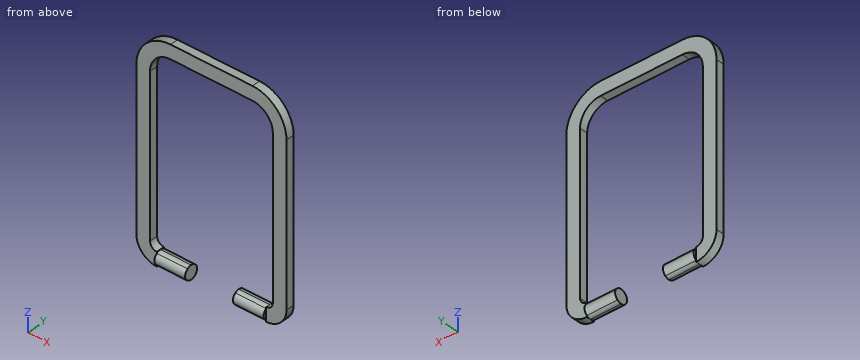
from build123d import *
from build123d import SkipClean  # not in build123d's __all__

# Parameters (mm, degrees)
F1_DEPTH = 1.2
F3_DEPTH = 4.5
F4_DEPTH = 4.5
F6_DEPTH = 4.5
F7_DEPTH = 4.5


with BuildPart() as f1:
    # F0 (on Front) → F1 (new body)
    with BuildSketch(Plane.XZ):
        with BuildLine():
            Line((4.75, 0), (-7.25, 0))
            ThreePointArc((-7.25, 0), (-10.7855339059, -1.4644660941), (-12.25, -5))
            Line((-12.25, -5), (-12.25, -28))
            ThreePointArc((-12.25, -28), (-11.3713203436, -30.1213203436), (-9.25, -31))
            Line((-9.25, -31), (-4.75, -31))
            Line((-4.75, -31), (-4.75, -29))
            Line((-4.75, -29), (-9.25, -29))
            ThreePointArc((-9.25, -29), (-9.9571067812, -28.7071067812), (-10.25, -28))
            Line((-10.25, -28), (-10.25, -5))
            ThreePointArc((-10.25, -5), (-9.3713203436, -2.8786796564), (-7.25, -2))
            Line((-7.25, -2), (4.75, -2))
            ThreePointArc((4.75, -2), (6.8713203436, -2.8786796564), (7.75, -5))
            Line((7.75, -5), (7.75, -28))
            ThreePointArc((7.75, -28), (7.4571067812, -28.7071067812), (6.75, -29))
            Line((6.75, -29), (2.25, -29))
            Line((2.25, -29), (2.25, -31))
            Line((2.25, -31), (6.75, -31))
            ThreePointArc((6.75, -31), (8.8713203436, -30.1213203436), (9.75, -28))
            Line((9.75, -28), (9.75, -5))
            ThreePointArc((9.75, -5), (8.2855339059, -1.4644660941), (4.75, 0))
        make_face()
    extrude(amount=F1_DEPTH)

    # F2 (on face) → F3 (join)
    with BuildSketch(Plane.YZ.offset(-4.75)):
        with BuildLine():
            Line((-1.2, -30.8), (-1.2, -29.2))
            ThreePointArc((-1.2, -29.2), (-1.6, -30), (-1.2, -30.8))
        make_face()
        with BuildLine():
            ThreePointArc((-0.6, -29), (-0.916227766, -29.0513167019), (-1.2, -29.2))
            Line((-1.2, -29.2), (-1.2, -30.8))
            ThreePointArc((-1.2, -30.8), (-0.916227766, -30.9486832981), (-0.6, -31))
            ThreePointArc((-0.6, -31), (-0.283772234, -30.9486832981), (0, -30.8))
            Line((0, -30.8), (0, -29.2))
            ThreePointArc((0, -29.2), (-0.283772234, -29.0513167019), (-0.6, -29))
        make_face()
        with BuildLine():
            ThreePointArc((0.4, -30), (0.294427191, -29.5527864045), (0, -29.2))
            Line((0, -29.2), (0, -30.8))
            ThreePointArc((0, -30.8), (0.294427191, -30.4472135955), (0.4, -30))
        make_face()
    extrude(amount=-F3_DEPTH)

    # F2 (on face) → F4 (cut)
    with BuildSketch(Plane.YZ.offset(-4.75)):
        with BuildLine():
            Line((0, -29), (-0.6, -29))
            ThreePointArc((-0.6, -29), (-0.283772234, -29.0513167019), (0, -29.2))
            Line((0, -29.2), (0, -29))
        make_face()
        with BuildLine():
            Line((-0.6, -29), (-1.2, -29))
            Line((-1.2, -29), (-1.2, -29.2))
            ThreePointArc((-1.2, -29.2), (-0.916227766, -29.0513167019), (-0.6, -29))
        make_face()
        with BuildLine():
            ThreePointArc((0, -30.8), (-0.283772234, -30.9486832981), (-0.6, -31))
            Line((-0.6, -31), (0, -31))
            Line((0, -31), (0, -30.8))
        make_face()
        with BuildLine():
            ThreePointArc((-0.6, -31), (-0.916227766, -30.9486832981), (-1.2, -30.8))
            Line((-1.2, -30.8), (-1.2, -31))
            Line((-1.2, -31), (-0.6, -31))
        make_face()
    with SkipClean():  # cleaning this boolean's faces spoils the solid; the shape is the same uncleaned
        extrude(amount=-F4_DEPTH, mode=Mode.SUBTRACT)

    # F5 (on face) → F6 (join)
    with BuildSketch(Plane(origin=(2.25, 0, 0), x_dir=(0, -1, 0), z_dir=(-1, 0, 0))):
        with BuildLine():
            Line((1.2, -30.8), (1.2, -29.2))
            ThreePointArc((1.2, -29.2), (0.916227766, -29.0513167019), (0.6, -29))
            ThreePointArc((0.6, -29), (0.283772234, -29.0513167019), (0, -29.2))
            Line((0, -29.2), (0, -30.8))
            ThreePointArc((0, -30.8), (0.283772234, -30.9486832981), (0.6, -31))
            ThreePointArc((0.6, -31), (0.916227766, -30.9486832981), (1.2, -30.8))
        make_face()
        with BuildLine():
            Line((0, -30.8), (0, -29.2))
            ThreePointArc((0, -29.2), (-0.4, -30), (0, -30.8))
        make_face()
        with BuildLine():
            ThreePointArc((1.6, -30), (1.494427191, -29.5527864045), (1.2, -29.2))
            Line((1.2, -29.2), (1.2, -30.8))
            ThreePointArc((1.2, -30.8), (1.494427191, -30.4472135955), (1.6, -30))
        make_face()
    extrude(amount=-F6_DEPTH)

    # F5 (on face) → F7 (cut)
    with BuildSketch(Plane(origin=(2.25, 0, 0), x_dir=(0, -1, 0), z_dir=(-1, 0, 0))):
        with BuildLine():
            ThreePointArc((0, -29.2), (0.283772234, -29.0513167019), (0.6, -29))
            Line((0.6, -29), (0, -29))
            Line((0, -29), (0, -29.2))
        make_face()
        with BuildLine():
            Line((1.2, -29.2), (1.2, -29))
            Line((1.2, -29), (0.6, -29))
            ThreePointArc((0.6, -29), (0.916227766, -29.0513167019), (1.2, -29.2))
        make_face()
        with BuildLine():
            Line((0, -31), (0.6, -31))
            ThreePointArc((0.6, -31), (0.283772234, -30.9486832981), (0, -30.8))
            Line((0, -30.8), (0, -31))
        make_face()
        with BuildLine():
            Line((1.2, -31), (1.2, -30.8))
            ThreePointArc((1.2, -30.8), (0.916227766, -30.9486832981), (0.6, -31))
            Line((0.6, -31), (1.2, -31))
        make_face()
    with SkipClean():  # cleaning this boolean's faces spoils the solid; the shape is the same uncleaned
        extrude(amount=-F7_DEPTH, mode=Mode.SUBTRACT)


solid = f1.part
Could you check a few things on this model? Use its own coordinates, in mm. Coordinates: 2 decimals unless noted, no trailing zeros. Loops run counter-clockwise (first coordinate to the right, second up) from the corner with the lowest first, then second, coordinate; pieces in that order, holes last.
1. Imagine slicing it at B-B (z = -10.5). Please give me the cut outline in (x, y), and give its area (3 significant figures).
2. For P1, Ø8, axis at x = -9.5, z = -19.5, coming from the -Y side; P2, Ø0.6, axis at y = -0.5, z = -29.5, coming from the -X side, each with a flat end and sliding along its axis, tell me the tip position at first contact or that it passes through.
3. Imagine slicing it at D-D (x = 0). Please give me the cut outline in (y, z).
4. I need wall thicknesses on L1, parallel to X at y = -0.55, z = -18; L2, parallel to Z at x = -2.75, y = -0.1; L3, parallel to X at y = -0.7, z = -28.5. Which ranges of each line are inside material? Lowest first, please.
5. Imagine slicing it at C-C (x = 6). Please give me the cut outline in (y, z).
6. Imagine slicing it at A-A (x = -6.25). Please give me the cut outline in (y, z).
Computed values:
1. outline: (-12.25, -1.2) - (-10.25, -1.2) - (-10.25, 0) - (-12.25, 0) - close; (7.75, -1.2) - (9.75, -1.2) - (9.75, 0) - (7.75, 0) - close
1. area: 4.80 mm2
2. P1: stops at y = -1.2
2. P2: stops at x = -12
3. outline: (-1.2, -2) - (0, -2) - (0, 0) - (-1.2, 0) - close
4. L1: x = -12.25 to -10.25, 7.75 to 9.75
4. L2: z = -2 to 0
4. L3: x = -12.21 to -10.12, 7.62 to 9.71
5. outline: circle Ø2 at (-0.6, -30); (-1.2, -2.27) - (0, -2.27) - (0, -0.16) - (-1.2, -0.16) - close
6. outline: circle Ø2 at (-0.6, -30); (-1.2, -2) - (0, -2) - (0, 0) - (-1.2, 0) - close
